Geometry check sheet. Reference: the model listing, model coordinates, mm. Face numbers are marked on the shaded views. A direction names the side the tool comes from. Give positions to 0.01 mm unless a question says otherwise; leave off trailing zeros. Loops run counter-clockwise (first coordinate to the right, second up) from the corner with the lowest first, then second, coordinate; pieces in that order, holes last. Notation, with made-up numbers: (57.25, -37) -> (87.25, -37) arc R28 cw to (87.25, -17) -> close; hole circle Ø10 at (75, 50.25). An arc over 180 degrees is marked (long way). One line per item, written item: value. Start each with the question number.
(1) Sectioned sample at A-A, the plane x = 0. Record the cut outline in (y, z).
(2) Tool access check on the marked faces 4, 5 and 6. Record the directions out of +Z, -Z, +X, -X, +Y, -Y that give a thin tool (end or side, any length) a straight path to the whole face; none if there is none.
(3) Sectioned sample at C-C, the plane z = 38. State how many separate pieces and enclosed holes the cut face has, then the cut area to 3 significant figures.
(4) Draft check along Z on the marked faces 1, 2 and 3. Enter one of: pulls with the +Z half, pulls with the -Z half, needs draft (parallel to the pull), parting line crosses it, or undercut.
(5) Gauge pin test, flat ends, axial feed: pin 1 Ø12 at (y, z) = (7, 12.5) entering from -X; pin 2 Ø3 at (y, z) = (25.5, 35) entering from +X (3 decimals); pin 3 Ø14.5 at (x, z) = (20, -34.64) entering from -Y; pin 4 Ø12 at (x, y) = (-10, 33) entering from -Z. Record the tip position at first contact, or that the pin passes through.
(6) Sectioned sample at B-B, the plane y = 24. Record the cut outline in (x, z), then the cut area to 3 significant figures.
(7) Scan lines: line 1 along Z through (x, y) = (0, 17); line 2 along Z through (x, y) = (20, 8); line 3 along Y through (x, z) = (-29, 23). Record each from-to range of solid material in increasing order. Write a range as from..to.
from build123d import *

# Parameters (mm, degrees)
SKETCH_2_R          = 5.5
CUT_EXTRUDE_1_DEPTH = 75.204110398


with BuildPart() as part:
    # 草图1 → 旋转1 (revolve)
    with BuildSketch(Plane.XY, mode=Mode.PRIVATE) as revolve_1_sk:
        with BuildLine():
            ThreePointArc((-25, 22.5), (-21.464466094, 23.964466094), (-20, 27.5))
            Line((-20, 27.5), (-20, 40.5))
            Line((-20, 40.5), (-18, 42.5))
            Line((-18, 42.5), (-10, 42.5))
            Line((-10, 42.5), (-10, 0))
            Line((-10, 0), (-30, 0))
            Line((-30, 0), (-30, 2.5))
            Line((-30, 2.5), (-50, 2.5))
            Line((-50, 2.5), (-50, 20.5))
            Line((-50, 20.5), (-48, 22.5))
            Line((-48, 22.5), (-25, 22.5))
        make_face()
        with BuildLine():
            Line((30, 0), (30, 2.5))
            Line((30, 2.5), (50, 2.5))
            Line((50, 2.5), (50, 20.5))
            Line((50, 20.5), (48, 22.5))
            Line((48, 22.5), (25, 22.5))
            ThreePointArc((25, 22.5), (21.464466094, 23.964466094), (20, 27.5))
            Line((20, 27.5), (20, 40.5))
            Line((20, 40.5), (18, 42.5))
            Line((18, 42.5), (10, 42.5))
            Line((10, 42.5), (10, 0))
            Line((10, 0), (30, 0))
        make_face()
    revolve(revolve_1_sk.sketch.rotate(Axis((0, -641.580774088, 0), (0, 1, 0)), 180), axis=Axis((0, -641.580774088, 0), (0, 1, 0)))

    # 草图2 → 切除-拉伸1 (cut, through all)
    with BuildSketch(Plane(origin=(0, 22.5, 0), x_dir=(1, 0, 0), z_dir=(0, 1, 0))):
        with Locations(Location((-40, 0, 0), (0, 0, 180))):
            Circle(SKETCH_2_R)
        with Locations(Location((-20, 34.641016151, 0), (0, 0, 180))):
            Circle(SKETCH_2_R)
        with Locations(Location((20, 34.641016151, 0), (0, 0, 180))):
            Circle(SKETCH_2_R)
        with Locations(Location((40, 0, 0), (0, 0, 180))):
            Circle(SKETCH_2_R)
        with Locations(Location((20, -34.641016151, 0), (0, 0, 180))):
            Circle(SKETCH_2_R)
        with Locations(Location((-20, -34.641016151, 0), (0, 0, 180))):
            Circle(SKETCH_2_R)
    extrude(amount=-CUT_EXTRUDE_1_DEPTH, mode=Mode.SUBTRACT)


solid = part.part
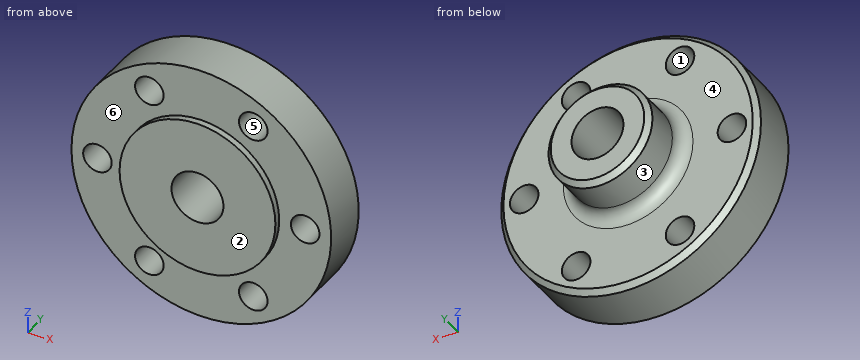
Calculated:
1. outline: (0, -30) -> (2.5, -30) -> (2.5, -50) -> (20.5, -50) -> (22.5, -48) -> (22.5, -25) arc R5 cw to (27.5, -20) -> (40.5, -20) -> (42.5, -18) -> (42.5, -10) -> (0, -10) -> close; (0, 10) -> (42.5, 10) -> (42.5, 18) -> (40.5, 20) -> (27.5, 20) arc R5 cw to (22.5, 25) -> (22.5, 48) -> (20.5, 50) -> (2.5, 50) -> (2.5, 30) -> (0, 30) -> close
2. face 4: +Y
2. face 5: +Y, -Y
2. face 6: -Y
3. separate pieces: 3
3. enclosed holes: 0
3. area: 945 mm2
4. face 1: undercut
4. face 2: needs draft
4. face 3: parting line crosses it
5. pin 1: stops at x = -49.58
5. pin 2: passes through
5. pin 3: stops at y = 2.5
5. pin 4: stops at z = -19.6
6. outline: circle Ø42.86 at (0, 0); hole circle Ø20 at (0, 0)
6. area: 1,130 mm2
7. line 1: z = -50..-10, 10..50
7. line 2: z = -45.83..-40.14, -29.14..29.14, 40.14..45.83
7. line 3: y = 2.5..22.5
